```python
from build123d import *

# Parameters (mm, degrees)
SKETCH3_R           = 2.4
REVOLVE1_ANGLE      = 120
SKETCH4_R           = 2.4
BOSS_EXTRUDE1_DEPTH = 20
SKETCH5_R           = 2.4
BOSS_EXTRUDE2_DEPTH = 20


with BuildPart() as part:
    # Sketch3 → Revolve1 (revolve)
    with BuildSketch(Plane.XY):
        with Locations((-201.5, 0)):
            Circle(SKETCH3_R)
    revolve(axis=Axis((0, 0, 0), (0, 1, 0)), revolution_arc=REVOLVE1_ANGLE)

    # Sketch4 → Boss-Extrude1 (add)
    with BuildSketch(Plane(origin=(0, 0, 0), x_dir=(-0.5000000000000043, 0, -0.8660254037844363), z_dir=(0.8660254037844362, 0, -0.5000000000000042))):
        with Locations(Location((-201.5, 0, 0), (0, 0, 180))):
            Circle(SKETCH4_R)
    extrude(amount=BOSS_EXTRUDE1_DEPTH)

    # Sketch5 → Boss-Extrude2 (add)
    with BuildSketch(Plane(origin=(0, 0, 0), x_dir=(-1, 0, 0), z_dir=(0, 0, -1))):
        with Locations((201.5, 0)):
            Circle(SKETCH5_R)
    extrude(amount=BOSS_EXTRUDE2_DEPTH)


solid = part.part
```
The listing builds one solid part. Answer for the finished solid, in the listing's coordinates (mm). Coordinates: 2 decimals unless noted, no trailing zeros. Loops run counter-clockwise (first coordinate to the right, second up) from the corner with the lowest first, then second, coordinate; pieces in that order, holes last. Notation, with made-up numbers: M 22,35.5 L 54,35.5 A15 ccw 54,44.5 Z; hole C 65,2.5 d11. An arc over 180 degrees is marked long. Answer as CSV lines item,"result". Start each with the question number.
(1) Given pin 1 (1 mm diameter, centred on x = -1.5, y = 1, fed in from -Z), flat-ended and moving along its own axis, determine where the tip first touches the part or whether it passes through.
(2) The part is cut by section A-A (y = 0). Give the vertices of the cut face in (x, z).
(3) Find the intervals of material crossed by L1, parallel to X at y = -0.8, z = 9.5; L2, parallel to Z at x = 43.5, y = -1.6; L3, parallel to Z at x = 105, y = -1.5, in increasing order. Write a range as [from, to].
Determined:
1,pin 1,"z = 199.15"
2,outline,"M -203.9,-20 L -199.1,-20 L -199.1,0 A199.1 cw 99.55,172.43 L 116.87,162.43 L 119.27,166.58 L 101.95,176.58 A203.9 ccw -203.9,0 Z"
3,L1,"[-203.54, -199.01]"
3,L2,"[194.92, 198.58]"
3,L3,"[169.89, 174.21]"
